Work out the finished part from the listing and answer in its coordinate system (mm). A direction names the side the tool comes from. Coordinates: 2 decimals unless noted, no trailing zeros. Order: outer loops, then holes, each group sorted by start corner. A loop starts at its lowest first (then second) coordinate and runs counter-clockwise, first axis right, second up. Notation, with made-up numbers: M 32.5,-18 L 83.5,-18 A6 ccw 83.5,-10 Z; hole C 29,50 d11. An arc over 180 degrees is marked long. Use a Markdown table: item, result. Add a question column.
from build123d import *

# Parameters (mm, degrees)
F0_R     = 1.778
F1_DEPTH = 5.08
F2_R     = 3.81
F2_R_2   = 1.778
F3_DEPTH = 6.35
F4_R     = 5.08
F5_R     = 1.016


# Not quite as in the source:
# - a feature names something its author has since deleted; it is built from what else it names


with BuildPart() as f1:
    # F0 (on Front) → F1 (new body)
    with BuildSketch(Plane.XZ):
        with BuildLine():
            ThreePointArc((5.0308613437, -0.7048646254), (5.0677004463, -0.353287683), (5.08, 0))
            ThreePointArc((5.08, 0), (5.0677004463, 0.353287683), (5.0308613437, 0.7048646254))
            ThreePointArc((5.0308613437, 0.7048646254), (4.3994090512, 2.54), (3.1258613437, 4.0044214139))
            ThreePointArc((3.1258613437, 4.0044214139), (2.54, 4.3994090512), (1.905, 4.7092860393))
            ThreePointArc((1.905, 4.7092860393), (0, 5.08), (-1.905, 4.7092860393))
            ThreePointArc((-1.905, 4.7092860393), (-2.54, 4.3994090512), (-3.1258613437, 4.0044214139))
            ThreePointArc((-3.1258613437, 4.0044214139), (-4.3994090512, 2.54), (-5.0308613437, 0.7048646254))
            ThreePointArc((-5.0308613437, 0.7048646254), (-5.08, 0), (-5.0308613437, -0.7048646254))
            ThreePointArc((-5.0308613437, -0.7048646254), (-4.3994090512, -2.54), (-3.1258613437, -4.0044214139))
            ThreePointArc((-3.1258613437, -4.0044214139), (-2.54, -4.3994090512), (-1.905, -4.7092860393))
            ThreePointArc((-1.905, -4.7092860393), (0, -5.08), (1.905, -4.7092860393))
            ThreePointArc((1.905, -4.7092860393), (2.54, -4.3994090512), (3.1258613437, -4.0044214139))
            ThreePointArc((3.1258613437, -4.0044214139), (4.3994090512, -2.54), (5.0308613437, -0.7048646254))
        make_face()
        Circle(F0_R, mode=Mode.SUBTRACT)
        with BuildLine():
            ThreePointArc((3.1258613437, 4.0044214139), (4.3994090512, 2.54), (5.0308613437, 0.7048646254))
            Line((5.0308613437, 0.7048646254), (6.9846726717, 2.1261920584))
            Line((6.9846726717, 2.1261920584), (8.7398771973, 4.1660886423))
            Line((8.7398771973, 4.1660886423), (7.9778771973, 5.4859113577))
            Line((7.9778771973, 5.4859113577), (5.3336726717, 4.9858079416))
            Line((5.3336726717, 4.9858079416), (3.1258613437, 4.0044214139))
        make_face()
        with BuildLine():
            Line((6.9846726717, -2.1261920584), (5.0308613437, -0.7048646254))
            ThreePointArc((5.0308613437, -0.7048646254), (4.3994090512, -2.54), (3.1258613437, -4.0044214139))
            Line((3.1258613437, -4.0044214139), (5.3336726717, -4.9858079416))
            Line((5.3336726717, -4.9858079416), (7.9778771973, -5.4859113577))
            Line((7.9778771973, -5.4859113577), (8.7398771973, -4.1660886423))
            Line((8.7398771973, -4.1660886423), (6.9846726717, -2.1261920584))
        make_face()
        with BuildLine():
            ThreePointArc((-1.905, 4.7092860393), (0, 5.08), (1.905, 4.7092860393))
            Line((1.905, 4.7092860393), (1.651, 7.112))
            Line((1.651, 7.112), (0.762, 9.652))
            Line((0.762, 9.652), (-0.762, 9.652))
            Line((-0.762, 9.652), (-1.651, 7.112))
            Line((-1.651, 7.112), (-1.905, 4.7092860393))
        make_face()
        with BuildLine():
            Line((1.651, -7.112), (1.905, -4.7092860393))
            ThreePointArc((1.905, -4.7092860393), (0, -5.08), (-1.905, -4.7092860393))
            Line((-1.905, -4.7092860393), (-1.651, -7.112))
            Line((-1.651, -7.112), (-0.762, -9.652))
            Line((-0.762, -9.652), (0.762, -9.652))
            Line((0.762, -9.652), (1.651, -7.112))
        make_face()
        with BuildLine():
            ThreePointArc((-5.0308613437, 0.7048646254), (-4.3994090512, 2.54), (-3.1258613437, 4.0044214139))
            Line((-3.1258613437, 4.0044214139), (-5.3336726717, 4.9858079416))
            Line((-5.3336726717, 4.9858079416), (-7.9778771973, 5.4859113577))
            Line((-7.9778771973, 5.4859113577), (-8.7398771973, 4.1660886423))
            Line((-8.7398771973, 4.1660886423), (-6.9846726717, 2.1261920584))
            Line((-6.9846726717, 2.1261920584), (-5.0308613437, 0.7048646254))
        make_face()
        with BuildLine():
            Line((-5.3336726717, -4.9858079416), (-3.1258613437, -4.0044214139))
            ThreePointArc((-3.1258613437, -4.0044214139), (-4.3994090512, -2.54), (-5.0308613437, -0.7048646254))
            Line((-5.0308613437, -0.7048646254), (-6.9846726717, -2.1261920584))
            Line((-6.9846726717, -2.1261920584), (-8.7398771973, -4.1660886423))
            Line((-8.7398771973, -4.1660886423), (-7.9778771973, -5.4859113577))
            Line((-7.9778771973, -5.4859113577), (-5.3336726717, -4.9858079416))
        make_face()
    extrude(amount=F1_DEPTH)

    # F2 (on face) → F3 (join)
    with BuildSketch(Plane.XZ.offset(5.08)):
        Circle(F2_R)
        Circle(F2_R_2, mode=Mode.SUBTRACT)
    extrude(amount=F3_DEPTH)

    # F4
    f4_edges = [f1.edges().sort_by_distance(p)[0] for p in [
        (1.651, -2.54, 7.112),
        (-1.651, -2.54, 7.112),
    ]]
    fillet(f4_edges, radius=F4_R)

    # F5
    f5_edges = [f1.edges().sort_by_distance(p)[0] for p in [
        (0.762, -2.54, 9.652),
        (-0.762, -2.54, 9.652),
    ]]
    fillet(f5_edges, radius=F5_R)


solid = f1.part
(1) Given P1, Ø2, axis at y = -1.5, z = 0, coming from the -X side; P2, Ø1, axis at y = -3.5, z = -5, coming from the -X side; P3, Ø1.5, axis at x = 7, y = -5.5, coming from the +Z side, each flat-ended and moving along its own axis, determine where each tip first touches the part or whether it passes through.
(2) A cutting plane is placed at C-C on x = 6.75. Write down the section's boundary in (y, z).
(3) Straight lines are drawn through the part: line 1 (Z direction, x = 0, y = -5); line 2 (Z direction, x = 0, y = -8.5); line 3 (Z direction, x = -3.5, y = -4.5). For each, find the intervals that lie inside material, in ascending order.
(4) The mould has two halves that part along Z. Classify faces 1 (the flat face through (-7.875, -2.504, 3.16)), 2 (the flat face through (8.364, -2.504, 4.817)), 3 (the flat face through (8.35, -2.5, -4.84)), 4 (the flat face through (7.875, -2.504, -3.16)): pulls with the +Z half, pulls with the -Z half, needs draft (parallel to the pull), parting line crosses it, or undercut.
(5) Which of the six approach directions +Z, -Z, +X, -X, +Y, -Y give full straight-line access (tool end or side, diameter ignored) to faces 5 (the flat face through (-5.994, -2.504, -1.406)), 6 (the flat face through (7.85, -2.5, 3.13)), 7 (the flat face through (-6.637, -2.504, 5.232)), 8 (the cylindrical face through (2.531, -2.504, -4.404))?
(6) A cutting plane is placed at D-D on x = -4.5. Write down the section's boundary in (y, z), plus the area to 3 significant figures.
(7) A cutting plane is placed at B-B on y = -6. Write down the section's boundary in (x, z), plus the area to 3 significant figures.
(8) A cutting plane is placed at A-A on x = -6.25. Write down the section's boundary in (y, z).
From the geometry:
| question | item | result |
|---|---|---|
| 1 | P1 | stops at x = -5.44 |
| 1 | P2 | stops at x = -8.55 |
| 1 | P3 | stops at z = 5.42 |
| 2 | outline | M -5.08,-5.25 L 0,-5.25 L 0,-1.96 L -5.08,-1.96 Z; M -5.08,1.96 L 0,1.96 L 0,5.25 L -5.08,5.25 Z |
| 3 | line 1 | z = -9.65 to -1.78, 1.78 to 9.65 |
| 3 | line 2 | z = -3.81 to -1.78, 1.78 to 3.81 |
| 3 | line 3 | z = -4.17 to 4.17 |
| 4 | face 1 | undercut |
| 4 | face 2 | pulls with the +Z half |
| 4 | face 3 | pulls with the -Z half |
| 4 | face 4 | undercut |
| 5 | face 5 | -X, +Y, -Y |
| 5 | face 6 | +X, +Y, -Y |
| 5 | face 7 | +Z, +Y, -Y |
| 5 | face 8 | -Z, +Y, -Y |
| 6 | outline | M -5.08,-4.62 L 0,-4.62 L 0,4.62 L -5.08,4.62 Z |
| 6 | area | 46.9 mm2 |
| 7 | outline | C 0,0 d7.62; hole C 0,0 d3.56 |
| 7 | area | 35.7 mm2 |
| 8 | outline | M -5.08,-5.16 L 0,-5.16 L 0,-1.59 L -5.08,-1.59 Z; M -5.08,1.59 L 0,1.59 L 0,5.16 L -5.08,5.16 Z |
